Could you check a few things on this model? Use its own coordinates, in mm. Round coordinates to 2 decimals unless told otherwise and drop trailing zeros. Loops run counter-clockwise (first coordinate to the right, second up) from the corner with the lowest first, then second, coordinate; pieces in that order, holes last. Notation, with made-up numbers: M -2,-2.5 L 54,-2.5 A25 ccw 54,11.5 Z; hole C 22.25,76.25 d5. An arc over 180 degrees is marked long. Answer in a Markdown table with one row per item.
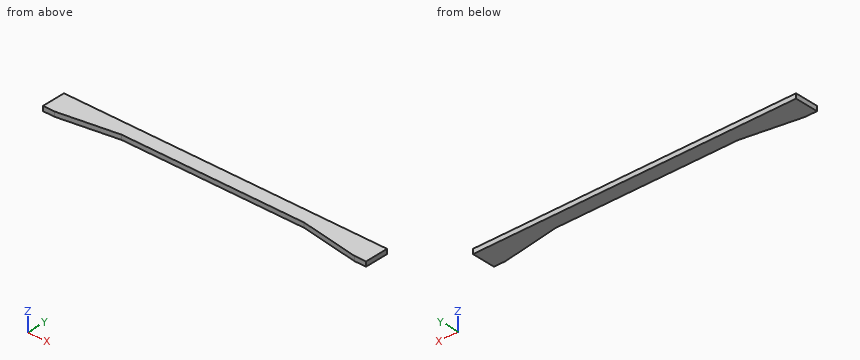
```python
from build123d import *

# Parameters (mm, degrees)
BOSS_EXTRUDE1_DEPTH = 4


with BuildPart() as part:
    # Sketch1 → Boss-Extrude1 (new body)
    with BuildSketch(Plane.XY):
        Polygon((0, 0), (-77.852222873, 0), (-127.75, -8), (-137.75, -8), (-137.75, 12), (0, 12), align=None)
    boss_extrude1 = extrude(amount=BOSS_EXTRUDE1_DEPTH)

    # Mirror1: Boss-Extrude1 across plane
    add(boss_extrude1.mirror(Plane(origin=(0, 0, 4), x_dir=(0, 0, 1), z_dir=(1, 0, 0))))


solid = part.part
```
1) I want a section at D-D, the plane x = 106. Please give me the cut outline in (y, z).
Computed:
| item | result |
|---|---|
| outline | M -4.51,0 L 12,0 L 12,4 L -4.51,4 Z |
2) I want a section at A-A, the plane y = -3.75. Please give me the cut outline in (x, z).
Computed:
| item | result |
|---|---|
| outline | M -137.75,0 L -101.24,0 L -101.24,4 L -137.75,4 Z; M 101.24,0 L 137.75,0 L 137.75,4 L 101.24,4 Z |
3) I want a section at C-C, the plane x = -53.5. Please give me the cut outline in (y, z), plus the area to 3 significant figures.
Computed:
| item | result |
|---|---|
| outline | M 0,0 L 12,0 L 12,4 L 0,4 Z |
| area | 48.0 mm² |
4) I need wall thicknesses on line 1 (Y direction, x = 27, z = 2.1); line 2 (Y direction, x = 109, z = 3.1). Which ranges of each line are inside material? Lowest first, please.
Computed:
| item | result |
|---|---|
| line 1 | y = 0 to 12 |
| line 2 | y = -4.99 to 12 |
5) I want a section at B-B, the plane z = 2.85. Please give me the cut outline in (x, y), plus the area to 3 significant figures.
Computed:
| item | result |
|---|---|
| outline | M -137.75,-8 L -127.75,-8 L -77.85,0 L 77.85,0 L 127.75,-8 L 137.75,-8 L 137.75,12 L -137.75,12 Z |
| area | 3,870 mm² |
6) Will this pin go through, and if not, where does the flat tip stop? P1, Ø2, axis at x = 91, z = 2.5, coming from the -Y side.
Computed:
| item | result |
|---|---|
| P1 | stops at y = -2.27 |
